Source: CAD feature listing. Evaluate the final solid. Frame: model axes, mm. Give positions to 0.01 mm unless a question says otherwise; leave off trailing zeros. Order: outer loops, then holes, each group sorted by start corner. A loop starts at its lowest first (then second) coordinate and runs counter-clockwise, first axis right, second up. Notation, with made-up numbers: M 46,9.25 L 105,9.25 A20 cw 105,34.25 Z; hole C -33,57.25 d5. An arc over 180 degrees is marked long. Return JSON: item names as keys, results as strings.
from build123d import *

# Parameters (mm, degrees)
EXTRUDE_1_DEPTH             = 10.5
FILLET_1_R                  = 0.3
FILLET_2_R                  = 2
HOLE_WIZARD_M41_D           = 3.3
HOLE_WIZARD_M41_CSINK_D     = 4.3
HOLE_WIZARD_M41_CSINK_ANGLE = 90


with BuildPart() as part:
    # Эскиз1 → Бобышка-Вытянуть1 (new body, symmetric)
    with BuildSketch(Plane.XY):
        with BuildLine():
            Line((-4, 0), (4, 0))
            Line((4, 0), (4, -0.8))
            Line((4, -0.8), (6.5, -0.8))
            Line((6.5, -0.8), (6.5, -1.6))
            ThreePointArc((6.5, -1.6), (4.386776199, -4.87777644), (1.5, -7.5))
            Line((1.5, -7.5), (-1.5, -7.5))
            ThreePointArc((-1.5, -7.5), (-4.386776199, -4.87777644), (-6.5, -1.6))
            Line((-6.5, -1.6), (-6.5, -0.8))
            Line((-6.5, -0.8), (-4, -0.8))
            Line((-4, -0.8), (-4, 0))
        make_face()
    extrude(amount=EXTRUDE_1_DEPTH, both=True)

    # Скругление1
    fillet_1_edges = [part.edges().sort_by_distance(p)[0] for p in [
        (6.5, -0.8, 0),
        (6.5, -1.6, 0),
        (-6.5, -1.6, 0),
        (-6.5, -0.8, 0),
        (-4, 0, 0),
        (4, 0, 0),
    ]]
    fillet(fillet_1_edges, radius=FILLET_1_R)

    # Скругление2
    fillet_2_edges = [part.edges().sort_by_distance(p)[0] for p in [
        (1.5, -7.5, 0),
        (-1.5, -7.5, 0),
    ]]
    fillet(fillet_2_edges, radius=FILLET_2_R)

    # Отверстие обработанное метчиком M41 (through all)
    with Locations(Plane(origin=(0, 0, 0), x_dir=(1, 0, 0), z_dir=(0, 1, 0))):
        with Locations((0, -4.5)):
            CounterSinkHole(HOLE_WIZARD_M41_D / 2, HOLE_WIZARD_M41_CSINK_D / 2, counter_sink_angle=HOLE_WIZARD_M41_CSINK_ANGLE)

    # Эскиз5 → Повернуть1 (revolve)
    with BuildSketch(Plane(origin=(0, 0, 0), x_dir=(0, 0, -1), z_dir=(1, 0, 0))):
        with BuildLine():
            Line((6.5, -4.3), (6.5, -8.3))
            ThreePointArc((6.5, -8.3), (4.5, -6.3), (6.5, -4.3))
        make_face()
    revolve(axis=Axis((0, -4.3, -6.5), (0, -1, 0)))


solid = part.part
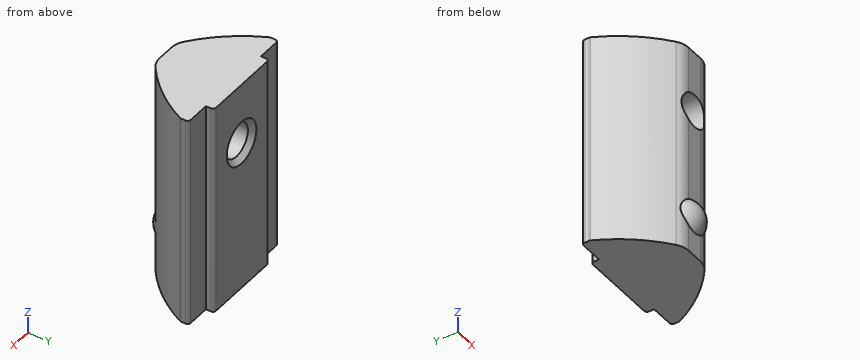
1. First-contact query: pin 1 (0.8 mm diameter, centred on x = 0, z = 8.5, fed in from -Y); pin 2 (2 mm diameter, centred on x = -4, z = 4.5, fed in from -Y); pin 3 (1.1 mm diameter, centred on x = 5, z = 4.5, fed in from +Y). Flat tips, straight axial feed; report the tip coordinate or a pass-through.
Evaluation:
{"pin 1": "stops at y = -7.5", "pin 2": "stops at y = -6.31", "pin 3": "stops at y = -0.8"}
2. Section query B-B (z = 4.5). Return loops of the section in (x, y).
Evaluation:
{"outline": "M -6.5,-1.53 A0.3 ccw -6.47,-1.66 A15 ccw -2.07,-7.09 A2 ccw -1.65,-7.33 L -1.65,-0.5 L -2.15,0 L -3.7,0 A0.3 ccw -4,-0.3 L -4,-0.8 L -6.2,-0.8 A0.3 ccw -6.5,-1.1 Z; M 1.65,-7.33 A2 ccw 2.07,-7.09 A15 ccw 6.47,-1.66 A0.3 ccw 6.5,-1.53 L 6.5,-1.1 A0.3 ccw 6.2,-0.8 L 4,-0.8 L 4,-0.3 A0.3 ccw 3.7,0 L 2.15,0 L 1.65,-0.5 Z"}
3. Section query C-C (y = -6.75). Return loops of the section in (x, z).
Evaluation:
{"outline": "M -2.49,-10.5 L 2.49,-10.5 L 2.49,10.5 L -2.49,10.5 Z; hole C 0,4.5 d3.3"}
4. Ray query, probe 1 along Z at (x, y) = (0, -3); probe 2 along Z at (x, y) = (1, -4.25); probe 3 along X at (y, z) = (-3.75, 4.5). Return the intervals inside material, ascending.
Evaluation:
{"probe 1": "z = -10.5 to 2.85, 6.15 to 10.5", "probe 2": "z = -10.5 to 3.19, 5.81 to 10.5", "probe 3": "x = -5.25 to -1.65, 1.65 to 5.25"}
5. Section query D-D (z = -4). Return loops of the section in (x, y), then the cut area to 3 significant figures.
Evaluation:
{"outline": "M -6.5,-1.53 A0.3 ccw -6.47,-1.66 A15 ccw -2.07,-7.09 A2 ccw -0.85,-7.5 L 0.85,-7.5 A2 ccw 2.07,-7.09 A15 ccw 6.47,-1.66 A0.3 ccw 6.5,-1.53 L 6.5,-1.1 A0.3 ccw 6.2,-0.8 L 4,-0.8 L 4,-0.3 A0.3 ccw 3.7,0 L -3.7,0 A0.3 ccw -4,-0.3 L -4,-0.8 L -6.2,-0.8 A0.3 ccw -6.5,-1.1 Z", "area": "69.1 mm^2"}
6. Section query A-A (x = 0). Return loops of the section in (y, z).
Evaluation:
{"outline": "M -7.5,-10.5 L 0,-10.5 L 0,2.35 L -0.5,2.85 L -7.5,2.85 L -7.5,-4.9 A2 ccw -7.5,-8.1 Z; M -7.5,6.15 L -0.5,6.15 L 0,6.65 L 0,10.5 L -7.5,10.5 Z"}
